from build123d import *

# Parameters (mm, degrees)
F2_DEPTH = 12.7
F3_DEPTH = 12.7
F4_R     = 15
F5_R     = 3.175
F6_DEPTH = 12.7


with BuildPart() as f2:
    # F0 (on Top) → F2 (new body)
    with BuildSketch(Plane.XY):
        with BuildLine():
            Line((88.9, 0), (88.9, 90.6961410425))
            ThreePointArc((88.9, 90.6961410425), (-127, 0), (88.9, -90.6961410425))
            Line((88.9, -90.6961410425), (88.9, 0))
        make_face()
        with BuildLine():
            Line((88.9, 0), (127, 0))
            ThreePointArc((127, 0), (117.0882146076, 49.1868884968), (88.9, 90.6961410425))
            Line((88.9, 90.6961410425), (88.9, 0))
        make_face()
        with BuildLine():
            ThreePointArc((88.9, -90.6961410425), (117.0882146076, -49.1868884968), (127, 0))
            Line((127, 0), (88.9, 0))
            Line((88.9, 0), (88.9, -90.6961410425))
        make_face()
    extrude(amount=F2_DEPTH)

    # F1 (on Top) → F3 (cut, through all)
    with BuildSketch(Plane.XY):
        Polygon((127, 52.5), (88.9, 19.177), (88.9, -19.177), (127, -52.5), align=None)
    extrude(amount=F3_DEPTH, mode=Mode.SUBTRACT)

    # F4
    f4_edges = [f2.edges().sort_by_distance(p)[0] for p in [
        (118.676596, -45.220189, 6.35),
        (118.676596, 45.220189, 6.35),
    ]]
    fillet(f4_edges, radius=F4_R)

    # F5 (on face) → F6 (cut, through all)
    with BuildSketch(Plane.XY.offset(12.7)):
        Circle(F5_R)
        with Locations((0, 25.4)):
            Circle(F5_R)
        with Locations((-21.9970452561, 12.7)):
            Circle(F5_R)
        with Locations((-21.9970452561, -12.7)):
            Circle(F5_R)
        with Locations((0, -25.4)):
            Circle(F5_R)
        with Locations((21.9970452561, -12.7)):
            Circle(F5_R)
        with Locations((21.9970452561, 12.7)):
            Circle(F5_R)
    extrude(amount=-F6_DEPTH, mode=Mode.SUBTRACT)


solid = f2.part
Verification items for the finished model (mm, model axes). A direction names the side the tool comes from. Give positions to 0.01 mm unless a question says otherwise; leave off trailing zeros. Write each loop counter-clockwise with the first axis right and the second up, starting at its lowest first coordinate (ties: lowest second). Pieces come first, ordered by that corner, then holes. Notation, with made-up numbers: (76, 24) - (115, 24) arc R15 ccw to (115, 44) - close; hole circle Ø9 at (6, 4). An arc over 180 degrees is marked (long way). Answer as CSV lines item,"result". Start each with the question number.
1. Set-up check for faces 1 (the face through (-19.064, 11.484, 6.439)), 2 (the face through (99.518, -28.464, 6.261)): record each of +Z, -Z, +X, -X, +Y, -Y from which the full face is reachable in a straight line by a thin tool's end or side.
2. Thickness scan on line 1 (Y direction, x = 0, z = 4.5) (3 decimals); line 2 (Y direction, x = 24.5, z = 2.75); line 3 (Y direction, x = 35.5, z = 2.25). Record the ranges inside material, lowest first.
3. Draft check along Y on faces 3 (the face through (99.82, 28.73, 6.26)), 4 (the face through (-7, 2, 12.7)). Enter one of: pulls with the +Y half, pulls with the -Y half, needs draft (parallel to the pull), parting line crosses it, or undercut.
4. Sectioned sample at D-D (x = -82). Record the boundary of the cut face in (y, z).
5. Sectioned sample at C-C (z = 7.25). Record the boundary of the cut face in (x, y) (3 decimals), then the cut area to 3 significant figures.
6. Depth check by flat-ended pin: pin 1 (4 mm diameter, centred on x = -22, y = 12.7, fed in from -Z); pin 2 (1 mm diameter, centred on y = -82.5, z = 3, fed in from +X); pin 3 (5 mm diameter, centred on y = 31.5, z = 9, fed in from +X); pin 4 (8 mm diameter, centred on x = 5, y = -101, fed in from -Z). Enter the tip coordinate at first touch or a pass-through.
7. Sectioned sample at A-A (x = 0). Record the boundary of the cut face in (y, z) (3 decimals).
8. Sectioned sample at B-B (y = 0). Record the boundary of the cut face in (x, z) (3 decimals).
Derived:
1,face 1,"+Z, -Z"
1,face 2,"+Z, -Z, +X"
2,line 1,"-127 to -28.575, -22.225 to -3.175, 3.175 to 22.225, 28.575 to 127"
2,line 2,"-124.61 to -14.65, -10.75 to 10.75, 14.65 to 124.61"
2,line 3,"-121.94 to 121.94"
3,face 3,"undercut"
3,face 4,"needs draft"
4,outline,"(-96.98, 0) - (96.98, 0) - (96.98, 12.7) - (-96.98, 12.7) - close"
5,outline,"(88.9, -19.177) - (88.9, 19.177) - (110.438, 38.015) arc R15 ccw to (114.031, 55.909) arc R127 ccw (long way) to (114.031, -55.909) arc R15 ccw to (110.438, -38.015) - close; hole circle Ø6.35 at (-21.997, -12.7); hole circle Ø6.35 at (-21.997, 12.7); hole circle Ø6.35 at (0, -25.4); hole circle Ø6.35 at (0, 0); hole circle Ø6.35 at (0, 25.4); hole circle Ø6.35 at (21.997, -12.7); hole circle Ø6.35 at (21.997, 12.7)"
5,area,"48,000 mm²"
6,pin 1,"through"
6,pin 2,"x = 96.98"
6,pin 3,"x = 105.85"
6,pin 4,"z = 0"
7,outline,"(-127, 0) - (-28.575, 0) - (-28.575, 12.7) - (-127, 12.7) - close; (-22.225, 0) - (-3.175, 0) - (-3.175, 12.7) - (-22.225, 12.7) - close; (3.175, 0) - (22.225, 0) - (22.225, 12.7) - (3.175, 12.7) - close; (28.575, 0) - (127, 0) - (127, 12.7) - (28.575, 12.7) - close"
8,outline,"(-127, 0) - (-3.175, 0) - (-3.175, 12.7) - (-127, 12.7) - close; (3.175, 0) - (88.9, 0) - (88.9, 12.7) - (3.175, 12.7) - close"
